Could you check a few things on this model? Use its own coordinates, in mm. Face numbers are marked on the shaded views. A direction names the side the tool comes from. Give positions to 0.01 mm unless a question says otherwise; leave off trailing zeros. Write each loop counter-clockwise with the first axis right and the second up, starting at its lowest first coordinate (ties: lowest second). Pieces come first, ordered by that corner, then holes. Notation, with made-up numbers: M -7,-8 L 50,-8 A29 cw 50,29 Z; hole C 37.5,62 d6. An arc over 180 degrees is marked long. Use one line per item in the form item = value.
from build123d import *


with BuildPart() as part:
    # Skica1 → Rotovat1 (revolve)
    with BuildSketch(Plane.XY):
        Polygon((-36.713340937, -44.25), (-56.713340937, -44.25), (-322.05, -19), (-340.05, -19), (-340.05, -17.3), (-341.55, -17.3), (-342.35, -18), (-347.05, -18), (-347.05, -15.5), (-345.05, -15.5), (-325.964213562, -15.5), (-324.964213562, -16.5), (-323.75, -16.5), (-323.75, -15.4), (-322.05, -15.4), (-322.05, -12.9), (-217.05, -23.4), (-217.05, -25.4), (-215.55, -25.4), (-215.55, -26.9), (-213.932233047, -26.9), (-212.632233047, -25.6), (-117.05, -29.4), (-117.05, -33.4), (-115.55, -33.4), (-115.55, -34.5), (-113.1872583, -34.5), (-112.099684413, -33.412426112), (-56.713340937, -36.8), (-27.213340937, -36.8), (-27.213340937, -40), (-33.813340937, -40), (-34.813340937, -39.3), (-36.713340937, -39.3), align=None)
    revolve(axis=Axis((-172.442437001, 0, 0), (1, 0, 0)))


solid = part.part
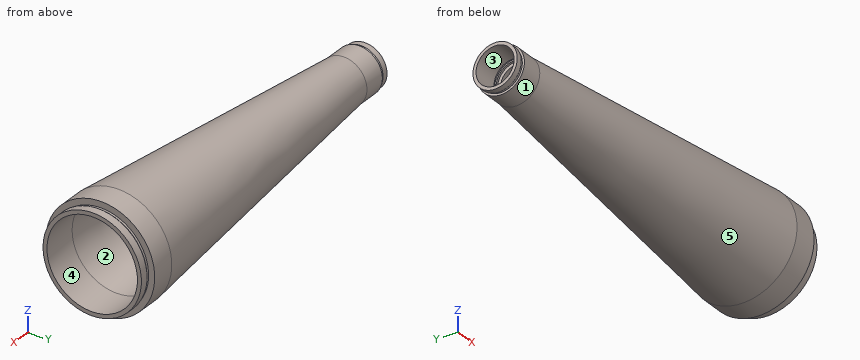
1) Thinking about a two-plate mould opening in Z: for the marked faces 3, 4 and 5, which applies, released by +Z, released by -Z, zero draft, split by the parting line, or undercut?
Checked values:
face_3 = undercut
face_4 = undercut
face_5 = split by the parting line
2) If I drill on L1, parallel to Y at x = -324.4, z = 0; L2, parallel to Y at x = -339, z = 0; L3, parallel to Z at x = -205, y = 10.5, over which ranges is the centre line in solid material (lowest first)?
Checked values:
L1 = -19 to -16.5, 16.5 to 19
L2 = -19 to -15.5, 15.5 to 19
L3 = -28.25 to -23.68, 23.68 to 28.25
3) For pin 1 Ø3 at (x, y) = (-70.5, 22) entering from +Z; pin 2 Ø4 at (x, z) = (-138.5, -17.5) entering from +Y; pin 3 Ø1 at (x, z) = (-283, 13.5) entering from -Y; pin 4 Ø16.5 at (y, z) = (-8, -7.5) entering from -X, each with a flat end and sliding along its axis, tell me the tip position at first contact or that it passes through.
Checked values:
pin_1 = 37.74
pin_2 = 33.03
pin_3 = -18.63
pin_4 = -347.05
4) For the marked faces 1 and 2, which set-ups out of +Z, -Z, +X, -X, +Y, -Y let a thin tool reach every point of the face, with its end or its side?
Checked values:
face_1 = -X
face_2 = +X
5) I want a section at A-A, the plane x = -290.5. Please give me the cut outline in (y, z) (3 decimals), plus the area to 3 significant figures.
Checked values:
outline = C 0,0 d44.005; hole C 0,0 d32.11
area = 711 mm2
6) I want a section at B-B, the plane x = -99. Please give me the cut outline in (y, z).
Checked values:
outline = C 0,0 d80.45; hole C 0,0 d68.43
